from build123d import *

# Parameters (mm, degrees)
SKETCH018_R      = 11
EXTRUDE016_DEPTH = 11
SKETCH015_W      = 33.86
SKETCH015_H      = 26.75
SKETCH015_R      = 1.65
EXTRUDE017_DEPTH = 1.6
SKETCH016_W      = 17
SKETCH016_H      = 12.75
EXTRUDE018_DEPTH = 4.3
SKETCH017_R      = 13.61
EXTRUDE015_DEPTH = 19.27


with BuildPart() as extrude_joystick_stick:
    # Sketch018 → Extrude016 (new body)
    with BuildSketch(Plane.XY):
        with Locations((16.975, 14)):
            Circle(SKETCH018_R)
    extrude(amount=EXTRUDE016_DEPTH)


with BuildPart() as extrude_joystick_stick_1:
    # Extrude016 placement: moved
    add(extrude_joystick_stick.part.moved(Location((0, 0, 20.87))))


with BuildPart() as extrude_joystick_base:
    # Sketch015 → Extrude017 (new body)
    with BuildSketch(Plane.XY):
        with Locations((16.93, 13.375)):
            Rectangle(SKETCH015_W, SKETCH015_H)
        with Locations((5, 22.88)):
            Circle(SKETCH015_R, mode=Mode.SUBTRACT)
        with Locations((31.01, 22.88)):
            Circle(SKETCH015_R, mode=Mode.SUBTRACT)
        with Locations((4.99, 3.31)):
            Circle(SKETCH015_R, mode=Mode.SUBTRACT)
        with Locations((31.01, 3.31)):
            Circle(SKETCH015_R, mode=Mode.SUBTRACT)
    extrude(amount=EXTRUDE017_DEPTH)


with BuildPart() as extrude_joystick_connector:
    # Sketch016 → Extrude018 (new body)
    with BuildSketch(Plane.XY):
        with Locations((-8.5, 13.875)):
            Rectangle(SKETCH016_W, SKETCH016_H)
    extrude(amount=EXTRUDE018_DEPTH)


with BuildPart() as extrude_joystick_connector_1:
    # Extrude018 placement: moved
    add(extrude_joystick_connector.part.moved(Location((0.1, 0, 1.6))))


with BuildPart() as fusion_joystick_connector:
    # Sketch017 → Extrude015 (new body)
    with BuildSketch(Plane.XY):
        with Locations((17.15, 13.61)):
            Circle(SKETCH017_R)
    extrude(amount=EXTRUDE015_DEPTH)


with BuildPart() as fusion_joystick_connector_1:
    # Extrude015 placement: moved
    add(fusion_joystick_connector.part.moved(Location((0, 0, 1.6))))

    # Fusion005: union Extrude_JoyStick_Stick, Extrude_JoyStick_base, Extrude_JoyStick_connector
    add(extrude_joystick_stick_1.part)
    add(extrude_joystick_base.part)
    add(extrude_joystick_connector_1.part)


with BuildPart() as fusion_joystick_connector_2:
    # Fusion005 placement: moved
    add(fusion_joystick_connector_1.part.moved(Location((53, 5, 5))))


solid = fusion_joystick_connector_2.part
Build history of the part. All positions in model axes, mm. A direction names the side the tool comes from. Coordinates: 2 decimals unless noted, no trailing zeros. Write each loop counter-clockwise with the first axis right and the second up, starting at its lowest first coordinate (ties: lowest second). Pieces come first, ordered by that corner, then holes. Notation, with made-up numbers: (57, 66.25) -> (103, 66.25) arc R20 cw to (103, 74.25) -> close; hole circle Ø1 at (-33, -4). An arc over 180 degrees is marked (long way). Use CSV: the item, a comma, the result in double quotes. Start each with the question number.
Q1. Flat gauge pins, fed straight in: pin 1 Ø4 at (x, y) = (84.01, 8.31) entering from +Z; pin 2 Ø2 at (x, y) = (58, 27.88) entering from +Z; pin 3 Ø2 at (x, z) = (46, 8) entering from -Y; pin 4 Ø1.8 at (y, z) = (12, 5.5) entering from -X. Where does each tip first touch, or does it go through?
Q2. Cut at A-A, the plane y = 9. List the corners of the cut face in (x, z).
Q3. Cut at D-D, the plane x = 64.5. List the corners of the cut face in (y, z).
Q4. Drill centre lines: probe 1 along Y at (x, z) = (58, 6.25); probe 2 along Z at (x, y) = (50.5, 19); probe 3 along Z at (x, y) = (60, 7). Where is each one in solid material? Low to high.
Q5. 3-axis set-ups, long thin cutter, end or side, ignore diameter. For faces 4 (the flat face through (70, 31.75, 6)), 5 (the flat face through (76.1, 9.6, 25.87)), 6 (the flat face through (53, 18, 6)): which of +Z, -Z, +X, -X, +Y, -Y reach the whole face in a straight line?
Q6. Cut at C-C, the plane y = 14. List the corners of the cut face in (x, z).
Q7. Cut at B-B, the plane x = 57.99. List the corners of the cut face in (y, z), then the cut area to 3 significant figures.
Q8. Pull direction Y, two halves, no side cores. Call faces 1 (the flat face through (44, 25.25, 9)), 2 (the cylindrical face through (85.584, 8.806, 5.789)), 3 (the cylindrical face through (75.05, 9.24, 31.29)): released by +Y, released by -Y, zero draft, split by the parting line, or undercut.
Checked values:
1,pin 1,"stops at z = 6.6"
1,pin 2,"passes through"
1,pin 3,"stops at y = 12.5"
1,pin 4,"stops at x = 53"
2,outline,"(53, 5) -> (56.49, 5) -> (56.49, 6.6) -> (53, 6.6) -> close; (59.49, 5) -> (82.51, 5) -> (82.51, 6.6) -> (79.79, 6.6) -> (79.79, 25.87) -> (74.56, 25.87) -> (74.56, 36.87) -> (65.39, 36.87) -> (65.39, 25.87) -> (60.51, 25.87) -> (60.51, 6.6) -> (59.49, 6.6) -> close; (85.51, 5) -> (86.86, 5) -> (86.86, 6.6) -> (85.51, 6.6) -> close"
3,outline,"(5, 5) -> (31.75, 5) -> (31.75, 6.6) -> (30.99, 6.6) -> (30.99, 25.87) -> (28.54, 25.87) -> (28.54, 36.87) -> (9.46, 36.87) -> (9.46, 25.87) -> (6.23, 25.87) -> (6.23, 6.6) -> (5, 6.6) -> close"
4,probe 1,"y = 5 to 6.66, 9.96 to 26.23, 29.53 to 31.75"
4,probe 2,"z = 6.6 to 10.9"
4,probe 3,"z = 5 to 6.6"
5,face 4,"-Z, +X, -X, +Y"
5,face 5,"+Z"
5,face 6,"-Z, -X, +Y, -Y"
6,outline,"(36.1, 6.6) -> (53, 6.6) -> (53, 5) -> (86.86, 5) -> (86.86, 6.6) -> (82.96, 6.6) -> (82.96, 25.87) -> (79.77, 25.87) -> (79.77, 36.87) -> (60.18, 36.87) -> (60.18, 25.87) -> (57.34, 25.87) -> (57.34, 6.6) -> (53.1, 6.6) -> (53.1, 10.9) -> (36.1, 10.9) -> close"
7,outline,"(5, 5) -> (6.66, 5) -> (6.66, 6.6) -> (5, 6.6) -> close; (9.96, 5) -> (26.23, 5) -> (26.23, 6.6) -> (24.72, 6.6) -> (24.72, 25.87) -> (12.5, 25.87) -> (12.5, 6.6) -> (9.96, 6.6) -> close; (29.53, 5) -> (31.75, 5) -> (31.75, 6.6) -> (29.53, 6.6) -> close"
7,area,"268 mm²"
8,face 1,"released by +Y"
8,face 2,"undercut"
8,face 3,"split by the parting line"
